Geometry check sheet. Reference: drawing and pictorial views, mm from the part's lowest x, y, z. A direction names the side the tool comes from. Round coordinates to 2 decimals unless told otherwise and drop trailing zeros. Write each loop counter-clockwise with the first axis right and the second up, starting at its lowest first coordinate (ties: lowest second). Pieces come first, ordered by that corner, then holes. Notation, with made-up numbers: M 32.25,78.5 L 39.25,78.5 A24 ccw 39.25,108.5 Z; hole C -9.75,-9 d9. An arc over 180 degrees is marked long. Use a Markdown table: item, result. Add a question column.
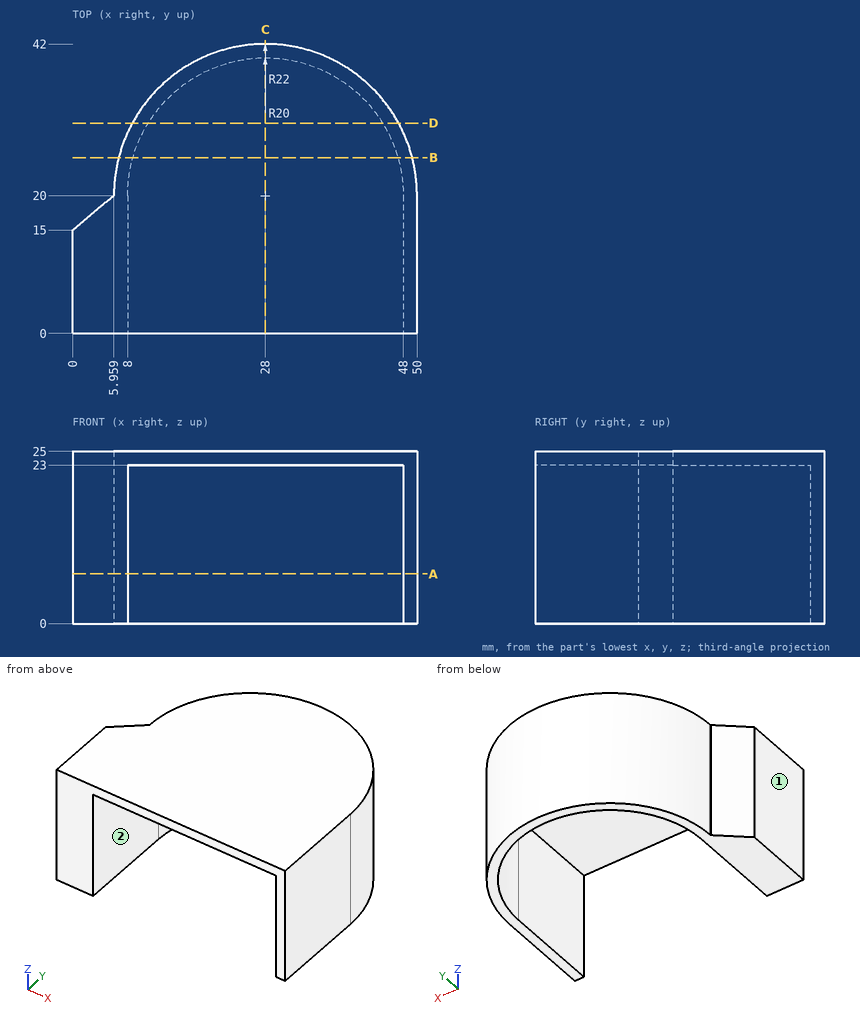
1. Depth check by flat-ended pin: pin 1 Ø6 at (y, z) = (34, 17.5) entering from -X; pin 2 Ø12 at (x, y) = (35, 27) entering from -Z; pin 3 Ø12 at (y, z) = (37.5, 11) entering from +X (1 decimal). Enter the tip coordinate at first touch or a pass-through.
2. Scan lines: line 1 along X through (y, z) = (6, 9); line 2 along Z through (x, y) = (42.5, 20); line 3 along X through (y, z) = (17, 14.5) (1 decimal). Record each from-to range of solid material in increasing order. Write a range as from..to.
3. Access from +Z, -Z, +X, -X, +Y, -Y to the whole of each face (thin tool, end or side, straight path). Record for the marked faces 1 and 2.
4. Cross-section at C-C on x = 28. Enter the section's corners in (y, z).
5. Cross-section at B-B on y = 25.5. Enter the section's corners in (x, z).
6. Cross-section at A-A on z = 7.25. Enter the section's corners in (x, y).
7. Cross-section at D-D on y = 30.5. Enter the section's corners in (x, z), plus the area to 3 significant figures.
Answer:
| question | item | result |
|---|---|---|
| 1 | pin 1 | stops at x = 8.95 |
| 1 | pin 2 | stops at z = 23 |
| 1 | pin 3 | stops at x = 46.8 |
| 2 | line 1 | x = 0..8, 48..50 |
| 2 | line 2 | z = 23..25 |
| 2 | line 3 | x = 2.4..8, 48..50 |
| 3 | face 1 | +Z, -Z, -X, +Y, -Y |
| 3 | face 2 | -Z, -Y |
| 4 | outline | M 0,23 L 40,23 L 40,0 L 42,0 L 42,25 L 0,25 Z |
| 5 | outline | M 6.7,0 L 8.77,0 L 8.77,23 L 47.23,23 L 47.23,0 L 49.3,0 L 49.3,25 L 6.7,25 Z |
| 6 | outline | M 0,0 L 8,0 L 8,20 A20 cw 48,20 L 48,0 L 50,0 L 50,20 A22 ccw 6,20 L 5.96,20 L 0,15 Z |
| 7 | outline | M 8.67,0 L 10.98,0 L 10.98,23 L 45.02,23 L 45.02,0 L 47.33,0 L 47.33,25 L 8.67,25 Z |
| 7 | area | 184 mm^2 |
